Autodesk Inventor part; units mm, degrees
ref_plane "Start Plane" through (0, 0, 0) normal (0, 0, 1) x (1, 0, 0)
ref_plane "End Plane" through (0, 0, 2881) normal (0, 0, 1) x (1, 0, 0)
ref_plane "YZ Plane" through (0, 0, 0) normal (1, 0, 0) x (0, 1, 0)
ref_plane "Start Plane" through (0, 0, 0) normal (0, 0, 1) x (1, 0, 0)
ref_plane "End Plane" through (0, 0, 2881) normal (0, 0, 1) x (1, 0, 0)
sketch "Sketch" plane through (0, 0, 0) normal (0, 0, 1) x (1, 0, 0)
  line L0 (-10, -14) -> (-10, 14)
  line L1 (-4, 20) -> (4, 20)
  line L2 (10, 14) -> (10, -14)
  line L3 (4, -20) -> (-4, -20)
  arc A0 (-10, -14) -> (-4, -20) centre (-4, -14) ccw
  arc A1 (10, 14) -> (4, 20) centre (4, 14) ccw
  arc A2 (-4, 20) -> (-10, 14) centre (-4, 14) ccw
  arc A3 (4, -20) -> (10, -14) centre (4, -14) ccw
  arc A4 (-4, 17) -> (-7, 14) centre (-4, 14) ccw
  line L4 (-4, 17) -> (4, 17)
  arc A5 (7, 14) -> (4, 17) centre (4, 14) ccw
  line L5 (7, 14) -> (7, -14)
  arc A6 (4, -17) -> (7, -14) centre (4, -14) ccw
  line L6 (4, -17) -> (-4, -17)
  arc A7 (-7, -14) -> (-4, -17) centre (-4, -14) ccw
  line L7 (-7, -14) -> (-7, 14)
  line L8 (0, 29.7397) -> (0, -29.7397) construction
  line L9 (-15.7397, 0) -> (15.7397, 0) construction
  dimension "d7" = 6
  dimension "d9" = 20
  dimension "d11" = 40
  dimension "d12" = 3
  dimension "d15" = 10
  dimension "d16" = 20
extrude "Body" add sketch "Sketch" along normal up to surface (2881 mm away) from surface at 0
sketch "Sketch3" plane through (0, 0, 0) normal (0, 0, 1) x (1, 0, 0)
  line L0 (0, 0) -> (10, 0)
ref_plane "Work Plane3" through (0, 0, 0) normal (0, -1, 0) x (1, 0, 0)
sketch "Sketch5" plane through (10, -14, 2881) normal (1, 0, 0) x (0, 0, -1)
  line L0 (0, 28) -> (0, 34)
  line L1 (0, 34) -> (32.0002, -6)
  line L2 (2881, -6) -> (0, -6)
  line L3 (0, -6) -> (0, 0)
  line L4 (0, 28) -> (0, 0)
  point P0 (2881, 14)
  dimension "d19" = 38.66
extrude "Extrusion2" cut sketch "Sketch5" against normal through all
sketch "Sketch4" plane through (0, 0, 0) normal (0, -1, 0) x (1, 0, 0)
  line L0 (-2, 0) -> (12, 0)
  line L1 (-2, 2881) -> (12, 2881)
  dimension "d18" = 2881
equation "\"d7\" = G_IR"
equation "\"d9\" = G_W"
equation "\"d11\" = G_H"
equation "\"d12\" = G_T"
equation "\"d15\" = 0.5 * d9"
equation "\"d16\" = 0.5 * d11"
equation "\"d3\" = G_L"
equation "\"G_W\" = 20"
equation "\"G_H\" = 40"
equation "\"G_T\" = 3"
equation "\"G_IR\" = 6"
equation "\"G_L\" = d18"
equation "\"G_OFFSET_START\" = 0"
equation "\"G_OFFSET_END\" = 0"
equation "\"d14\" = G_OFFSET_END + B_L"
equation "\"B_L\" = 2881"
properties part number "ISO 4019 - 40x20x3 - 2881" material "Steel, Mild"
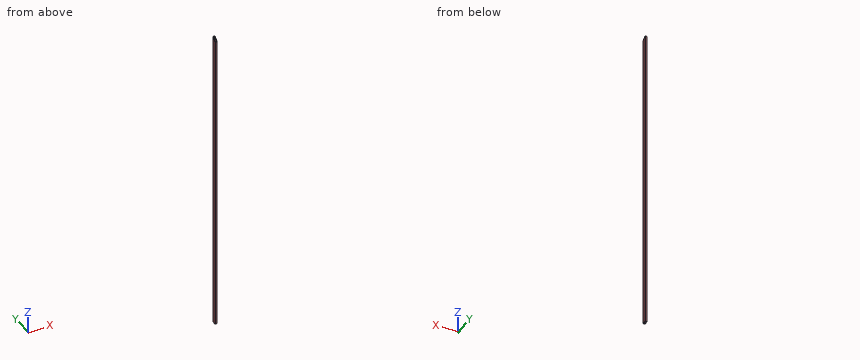
Geometry check sheet. Reference: the model listing, model coordinates, mm. Round coordinates to 2 decimals unless told otherwise and drop trailing zeros. Order: outer loops, then holes, each group sorted by start corner. A loop starts at its lowest first (then second) coordinate and runs counter-clockwise, first axis right, second up. Notation, with made-up numbers: (28, 15) - (73, 15) arc R26 cw to (73, 45) - close; hole circle Ø2 at (71, 88). An arc over 180 degrees is marked (long way). One line per question, with ' | ' between items. Start each with the question number.
(1) Sectioned sample at A-A on z = 2454.5. Record the cut outline in (x, y).
(2) Thickness scan on L1, parallel to Y at x = 1, z = 1291; L2, parallel to X at y = 2, z = 916.5; L3, parallel to Y at x = 5.5, z = 1609. Record the ranges inside material, lowest first. Write a range as [from, to].
(3) Sectioned sample at B-B on y = 3. Record the cut outline in (x, z).
(4) Depth check by flat-ended pin: pin 1 Ø10 at (x, y) = (2.5, 7.5) entering from +Z; pin 2 Ø5 at (x, y) = (4, 3) entering from -Z; pin 3 Ø5 at (y, z) = (-15.5, 1746) entering from +X. Enter the tip coordinate at first touch or a pass-through.
Conclusion:
1) outline: (-10, -14) arc R6 ccw to (-4, -20) - (4, -20) arc R6 ccw to (10, -14) - (10, 14) arc R6 ccw to (4, 20) - (-4, 20) arc R6 ccw to (-10, 14) - close; hole (-7, -14) arc R3 ccw to (-4, -17) - (4, -17) arc R3 ccw to (7, -14) - (7, 14) arc R3 ccw to (4, 17) - (-4, 17) arc R3 ccw to (-7, 14) - close
2) L1: y = [-20, -17], [17, 20] | L2: x = [-10, -7], [7, 10] | L3: y = [-19.81, -16.6], [16.6, 19.81]
3) outline: (-10, 0) - (-7, 0) - (-7, 2867.4) - (-10, 2867.4) - close; (7, 0) - (10, 0) - (10, 2867.4) - (7, 2867.4) - close
4) pin 1: stops at z = 2872.74 | pin 2: passes through | pin 3: stops at x = 10
